```python
from build123d import *

# Parameters (mm, degrees)
SKETCH1_R           = 70
SKETCH1_R_2         = 6
BOSS_EXTRUDE1_DEPTH = 20
SKETCH2_R           = 35
BOSS_EXTRUDE2_DEPTH = 35
SKETCH3_R           = 19
CUT_EXTRUDE1_DEPTH  = 56
FILLET1_R           = 6


with BuildPart() as part:
    # Sketch1 → Boss-Extrude1 (new body)
    with BuildSketch(Plane(origin=(0, 0, 0), x_dir=(1, 0, 0), z_dir=(0, 1, 0))):
        Circle(SKETCH1_R)
        with Locations((0, 55)):
            Circle(SKETCH1_R_2, mode=Mode.SUBTRACT)
        with Locations((55, 0)):
            Circle(SKETCH1_R_2, mode=Mode.SUBTRACT)
        with Locations((0, -55)):
            Circle(SKETCH1_R_2, mode=Mode.SUBTRACT)
        with Locations((-55, 0)):
            Circle(SKETCH1_R_2, mode=Mode.SUBTRACT)
    extrude(amount=BOSS_EXTRUDE1_DEPTH)

    # Sketch2 → Boss-Extrude2 (add)
    with BuildSketch(Plane(origin=(0, 20, 0), x_dir=(1, 0, 0), z_dir=(0, 1, 0))):
        Circle(SKETCH2_R)
    extrude(amount=BOSS_EXTRUDE2_DEPTH)

    # Sketch3 → Cut-Extrude1 (cut, through all)
    with BuildSketch(Plane(origin=(0, 55, 0), x_dir=(1, 0, 0), z_dir=(0, 1, 0))):
        Circle(SKETCH3_R)
    extrude(amount=-CUT_EXTRUDE1_DEPTH, mode=Mode.SUBTRACT)

    # Fillet1
    fillet1_edges = [part.edges().sort_by_distance(p)[0] for p in [
        (-35, 20, 0),
        (-35, 55, 0),
        (-70, 20, 0),
    ]]
    fillet(fillet1_edges, radius=FILLET1_R)


solid = part.part
```
The listing builds one solid part. Answer for the finished solid, in the listing's coordinates (mm). A direction names the side the tool comes from. Round coordinates to 2 decimals unless told otherwise and drop trailing zeros. Loops run counter-clockwise (first coordinate to the right, second up) from the corner with the lowest first, then second, coordinate; pieces in that order, holes last.
Q1. Find the intervals of material crossed by line 1 (X direction, y = 9, z = 0); line 2 (Z direction, x = 0, y = 15), in increasing order.
Q2. Given pin 1 Ø11 at (x, z) = (55, 0) entering from -Y; pin 2 Ø8 at (x, y) = (6, 13) entering from +Z; pin 3 Ø3 at (x, z) = (54.5, 26) entering from +Y; pin 4 Ø6 at (y, z) = (46.5, 3) entering from +X, each flat-ended and moving along its own axis, determine where each tip first touches the part or whether it passes through.
Q3. Section C-C, the plane y = 41 is taken. Determine the outline of the cut face in (x, z).
Q4. Which of the six approach directions +Z, -Z, +X, -X, +Y, -Y give full straight-line access (tool end or side, diameter ignored) to faces 1 (the face through (-1, 20, 42)), 2 (the face through (49, 10, 0))?
Q5. Section A-A, the plane z = 0 is taken. Determine the outline of the cut face in (x, y).
Q6. For a pull along Z with two mould halves and no side action, classify faces 3 (the face through (-1.301, 9.86, -49.143)), 4 (the face through (6, 55, 19)), 5 (the face through (-55.55, 6.902, 42.594)) as released by +Z, released by -Z, zero draft, split by the parting line, or undercut.
Q7. Section B-B, the plane y = 16 is taken. Determine the outline of the cut face in (x, z), then the cut area to 3 significant figures.
Completed:
1. line 1: x = -70 to -61, -49 to -19, 19 to 49, 61 to 70
1. line 2: z = -69.92 to -61, -49 to -19, 19 to 49, 61 to 69.92
2. pin 1: passes through
2. pin 2: stops at z = 69.97
2. pin 3: stops at y = 20
2. pin 4: stops at x = 35
3. outline: circle Ø70 at (0, 0); hole circle Ø38 at (0, 0)
4. face 1: +Y
4. face 2: +Y, -Y
5. outline: (-70, 0) - (-61, 0) - (-61, 20) - (-64, 20) arc R6 ccw to (-70, 14) - close; (-49, 0) - (-19, 0) - (-19, 55) - (-29, 55) arc R6 ccw to (-35, 49) - (-35, 26) arc R6 cw to (-41, 20) - (-49, 20) - close; (19, 0) - (49, 0) - (49, 20) - (41, 20) arc R6 cw to (35, 26) - (35, 49) arc R6 ccw to (29, 55) - (19, 55) - close; (61, 0) - (70, 0) - (70, 14) arc R6 ccw to (64, 20) - (61, 20) - close
6. face 3: undercut
6. face 4: zero draft
6. face 5: split by the parting line
7. outline: circle Ø139.31 at (0, 0); hole circle Ø12 at (-55, 0); hole circle Ø38 at (0, 0); hole circle Ø12 at (0, -55); hole circle Ø12 at (0, 55); hole circle Ø12 at (55, 0)
7. area: 13,700 mm2
